```python
from build123d import *

# Parameters (mm, degrees)
SKETCH1_R           = 10
SKETCH1_R_2         = 5
BOSS_EXTRUDE3_DEPTH = 20


with BuildPart() as part:
    # Sketch1 → Boss-Extrude3 (new body)
    with BuildSketch(Plane.XY):
        Polygon((-28.577015359, 8.156649179), (-28.577015359, 0.131238945), (-28.577015359, 0), (-28.577015359, -21.843350821), (21.422984641, -21.843350821), (21.422984641, -6.843350821), (36.422984641, -6.843350821), (36.422984641, 8.156649179), (51.422984641, 8.156649179), (51.422984641, 18.156649179), (6.422984641, 48.156649179), (-28.577015359, 48.156649179), (-28.577015359, 18.156649179), (-18.577015359, 18.156649179), (-18.577015359, 8.156649179), align=None)
        with Locations((1.422984641, -1.843350821)):
            Circle(SKETCH1_R, mode=Mode.SUBTRACT)
        with Locations((1.422984641, 33.156649179)):
            Circle(SKETCH1_R_2, mode=Mode.SUBTRACT)
    extrude(amount=BOSS_EXTRUDE3_DEPTH)


solid = part.part
```
The model under review builds one solid part; all positions refer to its coordinate system, in mm. A direction names the side the tool comes from. Round coordinates to 2 decimals unless told otherwise and drop trailing zeros. Loops run counter-clockwise (first coordinate to the right, second up) from the corner with the lowest first, then second, coordinate; pieces in that order, holes last. Notation, with made-up numbers: (-32, 31.25) - (-6, 31.25) arc R19 cw to (-6, 54.25) - close; hole circle Ø11 at (23.5, 40). An arc over 180 degrees is marked (long way). Write each question's results on one line, items separated by ' | '. Start each with the question number.
Q1. Take a section at A-A on x = -22.5. Give the boundary of the cut face in (y, z), plus the area to 3 significant figures.
Q2. Take a section at B-B on y = 4. Give the boundary of the cut face in (x, z).
Q3. Insertion check: P1, Ø6, axis at x = 1.42, y = 33.16, coming from the -Z side; P2, Ø4.5, axis at x = 46, z = 9, coming from the -Y side; P3, Ø4.5, axis at y = -17.5, z = 12, coming from the +X side; P4, Ø7.5, axis at y = 1, z = 13.5, coming from the +X side. Each pin has a flat end and moves straight along its axis. Give the tip position at first contact, or say it passes through.
Q4. Tool access review of faces 5 (the flat face through (44, 8.157, 10)), 6 (the flat face through (-18.577, 13, 10)), 7 (the flat face through (-4, -21.843, 10)): name each direction out of +Z, -Z, +X, -X, +Y, -Y from which nothing blocks a thin tool from reaching the whole face with its end or side.
Q5. Wall thickness on line 1 along Y through (x, z) = (4, 10.5); line 2 along Y through (x, z) = (2.5, 17.75); line 3 along X through (y, z) = (12, 14.25): over which ranges is each line inside the solid? List them lowest first. Write a range as [from, to].
Q6. Draft analysis for pull direction Y (two halves, no side actions). For faces 1 (the flat face through (29, -6.843, 10)), 2 (the cylindrical face through (-0.745, -11.606, 9.86)), 3 (the flat face through (-28.577, 33, 10)), 4 (the flat face through (-11, 48.157, 10)), state which applies: pulls with the +Y half, pulls with the -Y half, needs draft (parallel to the pull), parting line crosses it, or undercut.
Q7. Take a section at D-D on y = -13. Give the boundary of the cut face in (x, z), plus the area to 3 significant figures.
Q8. Take a section at C-C on z = 1.5. Give the boundary of the cut face in (x, y).
Data:
1) outline: (-21.84, 0) - (8.16, 0) - (8.16, 20) - (-21.84, 20) - close; (18.16, 0) - (48.16, 0) - (48.16, 20) - (18.16, 20) - close | area: 1,200 mm²
2) outline: (-28.58, 0) - (-6.69, 0) - (-6.69, 20) - (-28.58, 20) - close; (9.54, 0) - (36.42, 0) - (36.42, 20) - (9.54, 20) - close
3) P1: passes through | P2: stops at y = 8.16 | P3: stops at x = 21.42 | P4: stops at x = 36.42
4) face 5: +Z, -Z, +X, -Y | face 6: +Z, -Z, -X | face 7: +Z, -Z, +X, -X, -Y
5) line 1: y = [-21.84, -11.51], [7.82, 28.87], [37.44, 48.16] | line 2: y = [-21.84, -11.79], [8.1, 28.27], [38.04, 48.16] | line 3: x = [-18.58, 51.42]
6) face 1: pulls with the -Y half | face 2: undercut | face 3: needs draft | face 4: pulls with the +Y half
7) outline: (-28.58, 0) - (21.42, 0) - (21.42, 20) - (-28.58, 20) - close | area: 1,000 mm²
8) outline: (-28.58, -21.84) - (21.42, -21.84) - (21.42, -6.84) - (36.42, -6.84) - (36.42, 8.16) - (51.42, 8.16) - (51.42, 18.16) - (6.42, 48.16) - (-28.58, 48.16) - (-28.58, 18.16) - (-18.58, 18.16) - (-18.58, 8.16) - (-28.58, 8.16) - close; hole circle Ø20 at (1.42, -1.84); hole circle Ø10 at (1.42, 33.16)
